Part model, mm, in its own coordinate system. A direction names the side the tool comes from. Coordinates: 2 decimals unless noted, no trailing zeros. Order: outer loops, then holes, each group sorted by start corner. A loop starts at its lowest first (then second) coordinate and runs counter-clockwise, first axis right, second up. Notation, with made-up numbers: M -33.75,-11.5 L 23.25,-11.5 A18 cw 23.25,15.5 Z; hole C 14.25,3.5 d3. An arc over 180 degrees is marked long. Answer in a Markdown table with one row per item. Add a question column.
from build123d import *

# Parameters (mm, degrees)
SKETCH007_R     = 1.5
PAD002_DEPTH    = 7.5
SKETCH008_W     = 17.891225
SKETCH008_H     = 7
POCKET005_DEPTH = 36.001
SKETCH009_R     = 1.5
POCKET006_DEPTH = 6.001
SKETCH010_R     = 3
POCKET007_DEPTH = 3


with BuildPart() as bottom001:
    # Sketch007 → Pad002 (new body, symmetric)
    with BuildSketch(Plane.YZ):
        with BuildLine():
            ThreePointArc((4, 0), (0, 4), (-4, 0))
            ThreePointArc((-8, -4), (-5.171573, -2.828427), (-4, 0))
            Line((-21, -4), (-8, -4))
            Line((-21, -10), (-21, -4))
            Line((15, -10), (-21, -10))
            Line((15, -4), (15, -10))
            Line((8, -4), (15, -4))
            ThreePointArc((4, 0), (5.171573, -2.828427), (8, -4))
        make_face()
        Circle(SKETCH007_R, mode=Mode.SUBTRACT)
    extrude(amount=PAD002_DEPTH, both=True)

    # Sketch008 (on Face4 of Pad002) → Pocket005 (cut, through all)
    with BuildSketch(Plane(origin=(0, -21, 0), x_dir=(0, 0, -1), z_dir=(0, -1, 0))):
        with Locations((-4.945612, 0)):
            Rectangle(SKETCH008_W, SKETCH008_H)
    extrude(amount=-POCKET005_DEPTH, mode=Mode.SUBTRACT)

    # Sketch009 (on Face16 of Pocket005) → Pocket006 (cut, through all)
    with BuildSketch(Plane(origin=(0, 0, -4), x_dir=(0, -1, 0), z_dir=(0, 0, 1))):
        with Locations((16, 0)):
            Circle(SKETCH009_R)
        with Locations((-10, 0)):
            Circle(SKETCH009_R)
    extrude(amount=-POCKET006_DEPTH, mode=Mode.SUBTRACT)

    # Sketch010 (on Face5 of Pocket006) → Pocket007 (cut)
    with BuildSketch(Plane(origin=(0, 0, -4), x_dir=(0, -1, 0), z_dir=(0, 0, 1))):
        with Locations((-10, 0)):
            Circle(SKETCH010_R)
        with Locations((16, 0)):
            Circle(SKETCH010_R)
    extrude(amount=-POCKET007_DEPTH, mode=Mode.SUBTRACT)


with BuildPart() as part_mirroring001:
    # Part__Mirroring001: instance of Bottom001
    add(bottom001.part.mirror(Plane(origin=(0, 0, 0), x_dir=(0, 1, 0), z_dir=(0, 0, 1))))


solid = part_mirroring001.part
(1) Drop flat-ended pins along their axis: P1, Ø3, axis at x = 6, y = -15, coming from the -Z side; P2, Ø7.5, axis at x = -0.5, y = -3, coming from the -Z side; P3, Ø3.5, axis at x = 0, y = 10, coming from the -Z side. Give the stop position or say it passes through.
(2) Pull direction Z, two halves, no side cores. Call faces 1 (the cylindrical face through (-5.53, -1.5, -0.07)), 2 (the cylindrical face through (0, -13, 5)), 3 (the cylindrical face through (5.47, -1.5, -0.07)), 4 (the flat face through (-5, 11, 4)): pulls with the +Z half, pulls with the -Z half, needs draft (parallel to the pull), parting line crosses it, or undercut.
(3) Slice it at B-B (x = 0). List the corners of the cut face in (y, z).
(4) 3-axis set-ups, long thin cutter, end or side, ignore diameter. For faces 5 (the flat face through (0, -3, 4)), 6 (the flat face through (6, -15, 4)), 7 (the flat face through (6, 11, 4)), 8 (the flat face through (7.5, -3, 6)), 9 (the flat face through (-1.3, 8.7, 7)): which of +Z, -Z, +X, -X, +Y, -Y reach the whole face in a straight line?
(5) Slice it at C-C (z = 6). List the corners of the cut face in (x, y), and give its area (3 significant figures).
(6) Slice it at A-A (y = -16). List the corners of the cut face in (x, z).
(7) Wall check: line 1 (X direction, y = -16, z = 8.85); line 2 (Y direction, x = -1.5, z = 4.5); line 3 (Z direction, x = 4.8, y = 0). Give the ranges that are in metal, low to high.
(8) Slice it at D-D (y = 0). List the corners of the cut face in (x, z).
Computed:
| question | item | result |
|---|---|---|
| 1 | P1 | stops at z = 4 |
| 1 | P2 | stops at z = -3.93 |
| 1 | P3 | stops at z = 7 |
| 2 | face 1 | undercut |
| 2 | face 2 | needs draft |
| 2 | face 3 | undercut |
| 2 | face 4 | pulls with the -Z half |
| 3 | outline | M -21,4 L -19,4 L -19,7 L -17.5,7 L -17.5,10 L -21,10 Z; M -14.5,7 L -13,7 L -13,4 L 7,4 L 7,7 L 8.5,7 L 8.5,10 L -14.5,10 Z; M 11.5,7 L 13,7 L 13,4 L 15,4 L 15,10 L 11.5,10 Z |
| 4 | face 5 | -Z, +Y, -Y |
| 4 | face 6 | -Z, +X, -X, -Y |
| 4 | face 7 | -Z, +X, -X, +Y |
| 4 | face 8 | +Z, -Z, +X, +Y, -Y |
| 4 | face 9 | -Z |
| 5 | outline | M -7.5,-21 L 7.5,-21 L 7.5,15 L -7.5,15 Z; hole C 0,-16 d6; hole C 0,10 d6 |
| 5 | area | 483 mm^2 |
| 6 | outline | M -7.5,4 L -3,4 L -3,7 L -1.5,7 L -1.5,10 L -7.5,10 Z; M 1.5,7 L 3,7 L 3,4 L 7.5,4 L 7.5,10 L 1.5,10 Z |
| 7 | line 1 | x = -7.5 to -1.5, 1.5 to 7.5 |
| 7 | line 2 | y = -21 to -18.6, -13.4 to 7.4, 12.6 to 15 |
| 7 | line 3 | z = -4 to -1.5, 1.5 to 10 |
| 8 | outline | M -7.5,-4 L -3.5,-4 L -3.5,-1.5 L -7.5,-1.5 Z; M -7.5,1.5 L -3.5,1.5 L -3.5,4 L 3.5,4 L 3.5,1.5 L 7.5,1.5 L 7.5,10 L -7.5,10 Z; M 3.5,-4 L 7.5,-4 L 7.5,-1.5 L 3.5,-1.5 Z |
